from build123d import *

# Parameters (mm, degrees)
CROQUIS1_W              = 10
CROQUIS1_H              = 60
SALIENTE_EXTRUIR1_DEPTH = 9.12
CROQUIS2_R              = 2.4
CORTAR_EXTRUIR1_DEPTH   = 62.507514988
CROQUIS4_R              = 1.5
CORTAR_EXTRUIR2_DEPTH   = 62.507514988
REDONDEO1_R             = 1


with BuildPart() as part:
    # Croquis1 → Saliente-Extruir1 (new body)
    with BuildSketch(Plane(origin=(0, 0, 0), x_dir=(1, 0, 0), z_dir=(0, 1, 0))):
        with Locations((-5, -30)):
            Rectangle(CROQUIS1_W, CROQUIS1_H)
    extrude(amount=SALIENTE_EXTRUIR1_DEPTH)

    # Croquis2 → Cortar-Extruir1 (cut, through all)
    with BuildSketch(Plane.ZY.offset(10)):
        with Locations((17.5, 3.79)):
            Circle(CROQUIS2_R)
        with Locations((9.5, 3.79)):
            Circle(CROQUIS2_R)
        with Locations((25.5, 3.79)):
            Circle(CROQUIS2_R)
    extrude(amount=-CORTAR_EXTRUIR1_DEPTH, mode=Mode.SUBTRACT)

    # Croquis4 → Cortar-Extruir2 (cut, through all)
    with BuildSketch(Plane(origin=(0, 9.12, 0), x_dir=(1, 0, 0), z_dir=(0, 1, 0))):
        with Locations(Location((-5, -3, 0), (0, 0, 270))):
            Circle(CROQUIS4_R)
        with Locations(Location((-5, -57, 0), (0, 0, 270))):
            Circle(CROQUIS4_R)
    extrude(amount=-CORTAR_EXTRUIR2_DEPTH, mode=Mode.SUBTRACT)

    # Redondeo1
    redondeo1_edges = [part.edges().sort_by_distance(p)[0] for p in [
        (0, 9.12, 30),
        (-5, 9.12, 0),
        (-10, 9.12, 30),
        (-5, 9.12, 60),
    ]]
    fillet(redondeo1_edges, radius=REDONDEO1_R)


solid = part.part
Work out the finished part from the listing and answer in its coordinate system (mm). Give positions to 0.01 mm unless a question says otherwise; leave off trailing zeros. Write each loop counter-clockwise with the first axis right and the second up, starting at its lowest first coordinate (ties: lowest second). Pieces come first, ordered by that corner, then holes.
Q1. The part is cut by section B-B on x = -5. Give the vertices of the cut face in (y, z), and give its area (3 significant figures).
Answer:
outline: (0, 0) - (8.12, 0) arc R1 ccw to (9.12, 1) - (9.12, 1.5) - (0, 1.5) - close; (0, 4.5) - (9.12, 4.5) - (9.12, 55.5) - (0, 55.5) - close; (0, 58.5) - (9.12, 58.5) - (9.12, 59) arc R1 ccw to (8.12, 60) - (0, 60) - close; hole circle Ø4.8 at (3.79, 9.5); hole circle Ø4.8 at (3.79, 17.5); hole circle Ø4.8 at (3.79, 25.5)
area: 438 mm2
Q2. The part is cut by section A-A on z = 57. Give the vertices of the cut face in (x, y).
Answer:
outline: (-10, 0) - (-6.5, 0) - (-6.5, 9.12) - (-9, 9.12) arc R1 ccw to (-10, 8.12) - close; (-3.5, 0) - (0, 0) - (0, 8.12) arc R1 ccw to (-1, 9.12) - (-3.5, 9.12) - close
Q3. Straight lines are drawn through the part: L1, parallel to X at y = 6.5, z = 57; L2, parallel to Z at x = -1.5, y = 2.5; L3, parallel to Z at x = -2, y = 2.25. For each, find the intervals that lie inside material, in ascending order.
Answer:
L1: x = -10 to -6.5, -3.5 to 0
L2: z = 0 to 7.48, 11.52 to 15.48, 19.52 to 23.48, 27.52 to 60
L3: z = 0 to 7.66, 11.34 to 15.66, 19.34 to 23.66, 27.34 to 60
Q4. For a pull along Y with two mould halves and no side action, classify faces 1 (the face through (-5.07, 2.871, 27.717)), 2 (the face through (-10, 4, 30)), 3 (the face through (-5, 9.12, 30)) as released by +Y, released by -Y, zero draft, split by the parting line, or undercut.
Answer:
face 1: undercut
face 2: zero draft
face 3: released by +Y
Q5. The part is cut by section D-D on x = -2.75. Give the vertices of the cut face in (y, z).
Answer:
outline: (0, 0) - (8.12, 0) arc R1 ccw to (9.12, 1) - (9.12, 59) arc R1 ccw to (8.12, 60) - (0, 60) - close; hole circle Ø4.8 at (3.79, 9.5); hole circle Ø4.8 at (3.79, 17.5); hole circle Ø4.8 at (3.79, 25.5)
Q6. The part is cut by section C-C on y = 5.5. Give the vertices of the cut face in (x, z), and give its area (3 significant figures).
Answer:
outline: (-10, 0) - (0, 0) - (0, 7.82) - (-10, 7.82) - close; (-10, 11.18) - (0, 11.18) - (0, 15.82) - (-10, 15.82) - close; (-10, 19.18) - (0, 19.18) - (0, 23.82) - (-10, 23.82) - close; (-10, 27.18) - (0, 27.18) - (0, 60) - (-10, 60) - close; hole circle Ø3 at (-5, 3); hole circle Ø3 at (-5, 57)
area: 485 mm2
